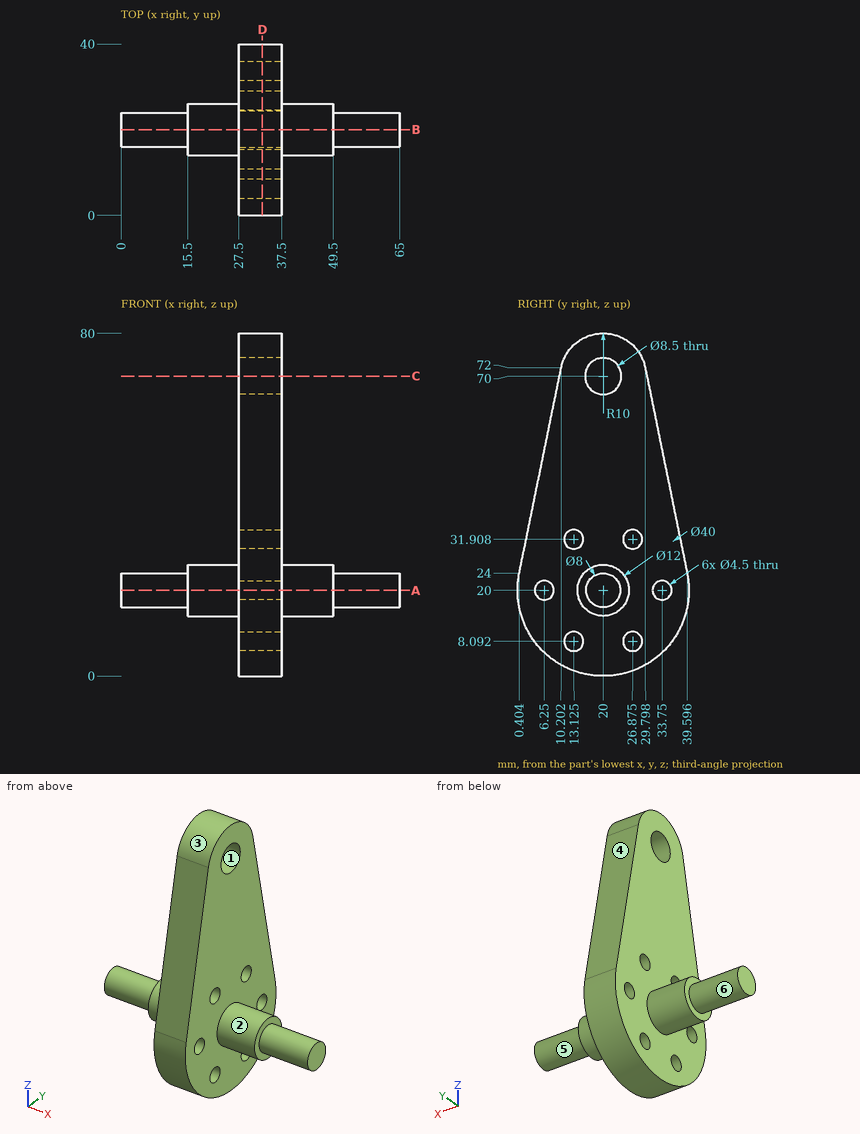
Job drawing, mm, ordinate dimensions from the low corner. One solid piece. A direction names the side the tool comes from. Give positions to 0.01 mm unless a question says otherwise; leave off trailing zeros. Loops run counter-clockwise (first coordinate to the right, second up) from the corner with the lowest first, then second, coordinate; pieces in that order, holes last.
Item 1: Slice it at D-D, the plane x = 33. List the corners of the cut face in (y, z) (3 decimals), and give its area (3 significant figures).
Answers follow:
outline: (0.404, 24) arc R20 ccw (long way) to (39.596, 24) - (29.798, 72) arc R10 ccw to (10.202, 72) - close; hole circle Ø4.5 at (6.25, 20); hole circle Ø4.5 at (13.125, 8.092); hole circle Ø4.5 at (13.125, 31.908); hole circle Ø8.5 at (20, 70); hole circle Ø4.5 at (26.875, 8.092); hole circle Ø4.5 at (26.875, 31.908); hole circle Ø4.5 at (33.75, 20)
area: 2,160 mm2
Item 2: Which spindle directions (+Z, -Z, +X, -X, +Y, -Y) get a long thin tool onto all of the face, cutting with end or side? Do the marked faces 4, 5 and 6. Say none if no direction does.
Answers follow:
face 4: +Z, +X, -X, +Y
face 5: +X
face 6: -X
Item 3: Slice it at A-A, the plane z = 20. List the corners of the cut face in (x, y).
Answers follow:
outline: (0, 16) - (15.5, 16) - (15.5, 14) - (27.5, 14) - (27.5, 8.5) - (37.5, 8.5) - (37.5, 14) - (49.5, 14) - (49.5, 16) - (65, 16) - (65, 24) - (49.5, 24) - (49.5, 26) - (37.5, 26) - (37.5, 31.5) - (27.5, 31.5) - (27.5, 26) - (15.5, 26) - (15.5, 24) - (0, 24) - close; (27.5, 0) - (37.5, 0) - (37.5, 4) - (27.5, 4) - close; (27.5, 36) - (37.5, 36) - (37.5, 40) - (27.5, 40) - close
Item 4: Drill centre lines: line 1 (Y direction, x = 30, z = 20); line 2 (X direction, y = 14, z = 67). Where is each one in solid material? Low to high.
Answers follow:
line 1: y = 0 to 4, 8.5 to 31.5, 36 to 40
line 2: x = 27.5 to 37.5
Item 5: Flat gauge pins, fed straight in: pin 1 (20 mm diameter, centred on y = 22.5, z = 39.5, fed in from +X); pin 2 (3 mm diameter, centred on y = 8, z = 66.5, fed in from -X). Where does each tip first touch, or does it go through?
Answers follow:
pin 1: stops at x = 37.5
pin 2: stops at x = 27.5
Item 6: Slice it at C-C, the plane z = 70. List the corners of the cut face in (x, y), and give its area (3 significant figures).
Answers follow:
outline: (27.5, 9.79) - (37.5, 9.79) - (37.5, 15.75) - (27.5, 15.75) - close; (27.5, 24.25) - (37.5, 24.25) - (37.5, 30.21) - (27.5, 30.21) - close
area: 119 mm2
Item 7: Pull direction Z, two halves, no side cores. Call the marked faces 1, 2 and 3: released by +Z, released by -Z, zero draft, split by the parting line, or undercut.
Answers follow:
face 1: undercut
face 2: split by the parting line
face 3: released by +Z
Item 8: Slice it at B-B, the plane y = 20. List the corners of the cut face in (x, z).
Answers follow:
outline: (0, 16) - (15.5, 16) - (15.5, 14) - (27.5, 14) - (27.5, 0) - (37.5, 0) - (37.5, 14) - (49.5, 14) - (49.5, 16) - (65, 16) - (65, 24) - (49.5, 24) - (49.5, 26) - (37.5, 26) - (37.5, 65.75) - (27.5, 65.75) - (27.5, 26) - (15.5, 26) - (15.5, 24) - (0, 24) - close; (27.5, 74.25) - (37.5, 74.25) - (37.5, 80) - (27.5, 80) - close
